Geometry check sheet. Reference: the model listing, model coordinates, mm. A direction names the side the tool comes from. Coordinates: 2 decimals unless noted, no trailing zeros. Loops run counter-clockwise (first coordinate to the right, second up) from the corner with the lowest first, then second, coordinate; pieces in that order, holes last.
from build123d import *

# Parameters (mm, degrees)
F1_DEPTH  = 6
F3_DEPTH  = 20
F5_DEPTH  = 40
F7_DEPTH  = 60
F9_DEPTH  = 2
F11_DEPTH = 2
F13_DEPTH = 2
F14_R     = 2.25
F15_DEPTH = 8
F16_R     = 2.25
F17_DEPTH = 8
F18_R     = 2.25
F19_DEPTH = 8
F20_R     = 3.75
F21_DEPTH = 2
F22_R     = 3.75
F23_DEPTH = 2
F24_R     = 3.75
F25_DEPTH = 2
F26_SIZE  = 3


with BuildPart() as f1:
    # F0 (on Top) → F1 (new body)
    with BuildSketch(Plane.XY):
        Polygon((0, 66), (0, 0), (66, 0), (66, 26), (26, 26), (26, 66), align=None)
    extrude(amount=F1_DEPTH)

    # F2 (on face) → F3 (join)
    with BuildSketch(Plane.XY.offset(6)):
        Polygon((6, 66), (0, 66), (0, 0), (66, 0), (66, 6), (6, 6), align=None)
    extrude(amount=F3_DEPTH)

    # F4 (on face) → F5 (join)
    with BuildSketch(Plane.XY.offset(26)):
        Polygon((6, 6), (6, 26), (0, 26), (0, 0), (26, 0), (26, 6), align=None)
    extrude(amount=F5_DEPTH)

    # F6 (on face) → F7 (join)
    with BuildSketch(Plane.XY.offset(6)):
        Polygon((13.29, 6), (16, 6), (18.71, 6), (18.71, 8), (13.29, 8), align=None)
        Polygon((6, 18.71), (6, 16), (6, 13.29), (8, 13.29), (8, 18.71), align=None)
    extrude(amount=F7_DEPTH)

    # F8 (on face) → F9 (join)
    with BuildSketch(Plane.XY.offset(6)):
        Polygon((66, 13.29), (66, 16), (66, 18.71), (26, 18.71), (26, 13.29), align=None)
        Polygon((18.71, 66), (16, 66), (13.29, 66), (13.29, 26), (18.71, 26), align=None)
    extrude(amount=F9_DEPTH)

    # F10 (on face) → F11 (join)
    with BuildSketch(Plane(origin=(0, 6, 0), x_dir=(-1, 0, 0), z_dir=(0, 1, 0))):
        Polygon((-66, 18.71), (-66, 16), (-66, 13.29), (-26, 13.29), (-26, 16), (-26, 18.71), align=None)
    extrude(amount=F11_DEPTH)

    # F12 (on face) → F13 (join)
    with BuildSketch(Plane.YZ.offset(6)):
        Polygon((66, 13.29), (66, 16), (66, 18.71), (26, 18.71), (26, 13.29), align=None)
    extrude(amount=F13_DEPTH)

    # F14 (on face) → F15 (cut, through all)
    with BuildSketch(Plane.XZ):
        with Locations((56, 16)):
            Circle(F14_R)
        with Locations((16, 46)):
            Circle(F14_R)
        with Locations((36, 16)):
            Circle(F14_R)
    extrude(amount=-F15_DEPTH, mode=Mode.SUBTRACT)

    # F16 (on face) → F17 (cut, through all)
    with BuildSketch(Plane(origin=(0, 0, 0), x_dir=(0, -1, 0), z_dir=(-1, 0, 0))):
        with Locations((-16, 56)):
            Circle(F16_R)
        with Locations((-46, 16)):
            Circle(F16_R)
        with Locations((-16, 36)):
            Circle(F16_R)
    extrude(amount=-F17_DEPTH, mode=Mode.SUBTRACT)

    # F18 (on face) → F19 (cut, through all)
    with BuildSketch(Plane(origin=(0, 0, 0), x_dir=(1, 0, 0), z_dir=(0, 0, -1))):
        with Locations((46, -16)):
            Circle(F18_R)
        with Locations((16, -56)):
            Circle(F18_R)
        with Locations((16, -36)):
            Circle(F18_R)
    extrude(amount=-F19_DEPTH, mode=Mode.SUBTRACT)

    # F20 (on face) → F21 (cut)
    with BuildSketch(Plane.XZ):
        with Locations((16, 46)):
            Circle(F20_R)
        with Locations((36, 16)):
            Circle(F20_R)
        with Locations((56, 16)):
            Circle(F20_R)
    extrude(amount=-F21_DEPTH, mode=Mode.SUBTRACT)

    # F22 (on face) → F23 (cut)
    with BuildSketch(Plane(origin=(0, 0, 0), x_dir=(0, -1, 0), z_dir=(-1, 0, 0))):
        with Locations((-16, 56)):
            Circle(F22_R)
        with Locations((-46, 16)):
            Circle(F22_R)
        with Locations((-16, 36)):
            Circle(F22_R)
    extrude(amount=-F23_DEPTH, mode=Mode.SUBTRACT)

    # F24 (on face) → F25 (cut)
    with BuildSketch(Plane(origin=(0, 0, 0), x_dir=(1, 0, 0), z_dir=(0, 0, -1))):
        with Locations((16, -56)):
            Circle(F24_R)
        with Locations((46, -16)):
            Circle(F24_R)
        with Locations((16, -36)):
            Circle(F24_R)
    extrude(amount=-F25_DEPTH, mode=Mode.SUBTRACT)

    # F26
    f26_edges = [f1.edges().sort_by_distance(p)[0] for p in [
        (33, 0, 0),
        (0, 33, 0),
        (0, 0, 33),
        (0, 26, 46),
        (0, 46, 26),
        (26, 0, 46),
        (46, 0, 26),
        (0, 13, 66),
        (13, 0, 66),
        (0, 66, 13),
        (13, 66, 0),
        (66, 0, 13),
        (66, 13, 0),
        (46, 26, 0),
        (26, 46, 0),
    ]]
    chamfer(f26_edges, length=F26_SIZE)


solid = f1.part
1) Section check A-A on y = 46. Record the cut outline in (x, z), and give its area (3 significant figures).
Data:
outline: (0, 3) - (3, 0) - (23, 0) - (26, 3) - (26, 6) - (18.71, 6) - (18.71, 8) - (13.29, 8) - (13.29, 6) - (6, 6) - (6, 13.29) - (8, 13.29) - (8, 13.75) - (2, 13.75) - (2, 12.25) - (0, 12.25) - close; (0, 19.75) - (2, 19.75) - (2, 18.25) - (8, 18.25) - (8, 18.71) - (6, 18.71) - (6, 26) - (3, 26) - (0, 23) - close
area: 242 mm2
2) Depth check by flat-ended pin: pin 1 (0.9 mm diameter, centred on x = 49, y = 4.5, fed in from +Z); pin 2 (3 mm diameter, centred on y = 39.5, z = 12.5, fed in from +X); pin 3 (5 mm diameter, centred on x = 54.5, y = 28, fed in from +Z); pin 4 (3.5 mm diameter, centred on x = 16, y = 36, fed in from -Z). Enter the tip coordinate at first touch or a pass-through.
Data:
pin 1: stops at z = 26
pin 2: stops at x = 8
pin 3: stops at z = 6
pin 4: passes through
3) Material ranges on probe 1 along Z at (x, y) = (36, 6.5); probe 2 along Y at (x, z) = (16, 4.9); probe 3 along Z at (x, y) = (56, 3.3), recorded low to high.
Data:
probe 1: z = 0 to 6, 13.29 to 13.75, 18.25 to 18.71
probe 2: y = 0 to 33.75, 38.25 to 53.75, 58.25 to 66
probe 3: z = 0 to 13.75, 18.25 to 26
4) Section check D-D on y = 16. Count the separate pieces of the cut face and the enclosed holes in it, and give its area (4 significant figures).
Data:
separate pieces: 4
enclosed holes: 0
area: 816.5 mm2
5) Mould release check, pull along X, two halves, no side actions. Record for faces 1 (the flat face through (66, 7, 14)), 2 (the flat face through (2, 2, 2)), 3 (the flat face through (46, 5, 26)), 4 (the flat face through (48, 18, 2)): +X half, -X half, draft (parallel to the pull), parting line (faces both ways), or undercut.
Data:
face 1: +X half
face 2: -X half
face 3: draft
face 4: undercut
6) Access from +Z, -Z, +X, -X, +Y, -Y to the whole of each face (thin tool, end or side, straight path). Record for faces 5 (the flat face through (7, 26, 16)), 6 (the flat face through (18, 2, 44)), 7 (the flat face through (7, 46, 18.71)), 8 (the flat face through (2, 14, 34)), 9 (the cylindrical face through (15.19, 59.66, 0.99)).
Data:
face 5: +Z, +X
face 6: -Y
face 7: +Z, +X, +Y
face 8: -X
face 9: -Z
7) Section check C-C on x = 51. Record the cut outline in (y, z), and give its area (3 significant figures).
Data:
outline: (0, 3) - (3, 0) - (23, 0) - (26, 3) - (26, 6) - (18.71, 6) - (18.71, 8) - (13.29, 8) - (13.29, 6) - (6, 6) - (6, 13.29) - (8, 13.29) - (8, 18.71) - (6, 18.71) - (6, 26) - (3, 26) - (0, 23) - close
area: 284 mm2
